```python
from build123d import *

# Parameters (mm, degrees)
SKETCH_1_R          = 13.85
EXTRUDE_1_DEPTH     = 32
SKETCH_2_R          = 2.5
EXTRUDE_2_DEPTH     = 2.5
SKETCH_3_R          = 8.5
EXTRUDE_3_DEPTH     = 4
EXTRUDE_START       = 18.5
SKETCH_4_R          = 2.5
EXTRUDE_4_DEPTH     = 18.5
CHAMFER_1_SIZE      = 2
CHAMFER_2_SIZE      = 1
SKETCH_5_R          = 1.35
CUT_EXTRUDE_1_DEPTH = 3


with BuildPart() as part:
    # 草图1 → 凸台-拉伸1 (new body)
    with BuildSketch(Plane(origin=(0, 0, 0), x_dir=(1, 0, 0), z_dir=(0, 1, 0))):
        with Locations(Location((0, 0, 0), (0, 0, 270))):
            Circle(SKETCH_1_R)
    extrude(amount=EXTRUDE_1_DEPTH)

    # 草图2 → 凸台-拉伸2 (add)
    with BuildSketch(Plane.XZ):
        with Locations(Location((0, 0, 0), (0, 0, 270))):
            Circle(SKETCH_2_R)
    extrude(amount=EXTRUDE_2_DEPTH)

    # 草图3 → 凸台-拉伸3 (add)
    with BuildSketch(Plane(origin=(0, 32, 0), x_dir=(1, 0, 0), z_dir=(0, 1, 0))):
        with Locations(Location((0, 0, 0), (0, 0, 270))):
            Circle(SKETCH_3_R)
    extrude(amount=EXTRUDE_3_DEPTH)

    # 草图4 → 凸台-拉伸4 (add)
    with BuildSketch(Plane(origin=(0, 36, 0), x_dir=(1, 0, 0), z_dir=(0, 1, 0)).offset(EXTRUDE_START)):
        with Locations(Location((0, 0, 0), (0, 0, 90))):
            Circle(SKETCH_4_R)
    extrude(amount=-EXTRUDE_4_DEPTH)

    # 倒角1
    chamfer_1_edges = [part.edges().sort_by_distance(p)[0] for p in [
        (0, 32, -13.85),
    ]]
    chamfer(chamfer_1_edges, length=CHAMFER_1_SIZE)

    # 倒角2
    chamfer_2_edges = [part.edges().sort_by_distance(p)[0] for p in [
        (0, 0, -13.85),
    ]]
    chamfer(chamfer_2_edges, length=CHAMFER_2_SIZE)

    # 草图5 → 切除-拉伸1 (cut)
    with BuildSketch(Plane.XZ):
        with Locations(Location((0, 8, 0), (0, 0, 270))):
            Circle(SKETCH_5_R)
        with Locations(Location((-9.5, 0, 0), (0, 0, 270))):
            Circle(SKETCH_5_R)
        with Locations(Location((0, -8, 0), (0, 0, 270))):
            Circle(SKETCH_5_R)
        with Locations(Location((9.5, 0, 0), (0, 0, 270))):
            Circle(SKETCH_5_R)
    extrude(amount=-CUT_EXTRUDE_1_DEPTH, mode=Mode.SUBTRACT)


solid = part.part
```
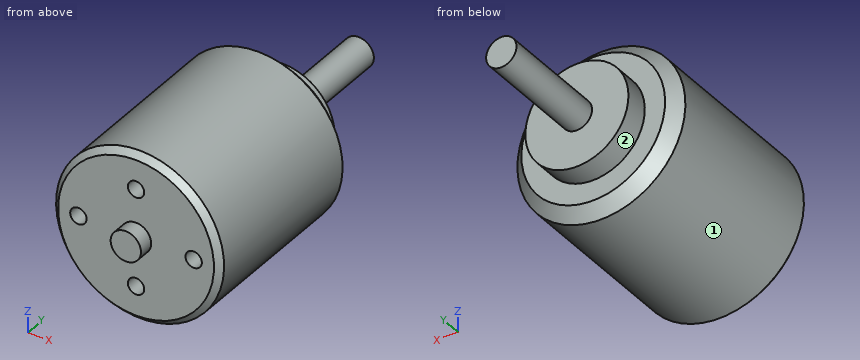
Source: CAD feature listing. Evaluate the final solid. Frame: model axes, mm. Face numbers are marked on the shaded views. A direction names the side the tool comes from. Round coordinates to 2 decimals unless told otherwise and drop trailing zeros. Loops run counter-clockwise (first coordinate to the right, second up) from the corner with the lowest first, then second, coordinate; pieces in that order, holes last.
(1) Section query B-B (z = 0). Output: boundary loops of the cut face in (x, y).
From the geometry:
outline: (-13.85, 1) - (-12.85, 0) - (-10.85, 0) - (-10.85, 3) - (-8.15, 3) - (-8.15, 0) - (-2.5, 0) - (-2.5, -2.5) - (2.5, -2.5) - (2.5, 0) - (8.15, 0) - (8.15, 3) - (10.85, 3) - (10.85, 0) - (12.85, 0) - (13.85, 1) - (13.85, 30) - (11.85, 32) - (8.5, 32) - (8.5, 36) - (2.5, 36) - (2.5, 54.5) - (-2.5, 54.5) - (-2.5, 36) - (-8.5, 36) - (-8.5, 32) - (-11.85, 32) - (-13.85, 30) - close
(2) Section query C-C (y = 49.5). Output: boundary loops of the cut face in (x, z), and give its area (3 significant figures).
From the geometry:
outline: circle Ø5 at (0, 0)
area: 19.6 mm2
(3) Contact query for flat-ended pins moving along their axis: pin 1 Ø5 at (y, z) = (8, 10.5) entering from -X; pin 2 Ø0.8 at (x, z) = (-0.5, 8) entering from -Y; pin 3 Ø2.5 at (x, z) = (9.5, 0) entering from +Y. Output: stop coordinate, or through.
From the geometry:
pin 1: stops at x = -11.31
pin 2: stops at y = 3
pin 3: stops at y = 36
(4) Section query A-A (x = 0). Output: boundary loops of the cut face in (y, z).
From the geometry:
outline: (-2.5, -2.5) - (0, -2.5) - (0, -6.65) - (3, -6.65) - (3, -9.35) - (0, -9.35) - (0, -12.85) - (1, -13.85) - (30, -13.85) - (32, -11.85) - (32, -8.5) - (36, -8.5) - (36, -2.5) - (54.5, -2.5) - (54.5, 2.5) - (36, 2.5) - (36, 8.5) - (32, 8.5) - (32, 11.85) - (30, 13.85) - (1, 13.85) - (0, 12.85) - (0, 9.35) - (3, 9.35) - (3, 6.65) - (0, 6.65) - (0, 2.5) - (-2.5, 2.5) - close
(5) Material intervals for probe 1 along X at (y, z) = (1.4, 0); probe 2 along X at (y, z) = (0.7, 0); probe 3 along X at (y, z) = (1.7, 8), sorted ascending.
From the geometry:
probe 1: x = -13.85 to -10.85, -8.15 to 8.15, 10.85 to 13.85
probe 2: x = -13.55 to -10.85, -8.15 to 8.15, 10.85 to 13.55
probe 3: x = -11.31 to -1.35, 1.35 to 11.31
(6) Access query for the marked faces 1 and 2. Directions: +Z, -Z, +X, -X, +Y, -Y. A direction counts if a zero-diameter tool reaches every point of the face in a straight line with its end or side. Return the directions, or none.
From the geometry:
face 1: +Y, -Y
face 2: +Y
(7) Section query D-D (y = 28.5). Output: boundary loops of the cut face in (x, z), and give its area (3 significant figures).
From the geometry:
outline: circle Ø27.7 at (0, 0)
area: 603 mm2
